Verification items for the finished model (mm, model axes). A direction names the side the tool comes from. Coordinates: 2 decimals unless noted, no trailing zeros. Write each loop counter-clockwise with the first axis right and the second up, starting at its lowest first coordinate (ties: lowest second). Pieces come first, ordered by that corner, then holes. Notation, with made-up numbers: (27, -29.5) -> (32, -29.5) arc R20 cw to (32, -22.5) -> close; hole circle Ø4 at (1, 24). An arc over 180 degrees is marked (long way). Write item = value, one per line. Start each with the question number.
(1) Gauge pin test, flat ends, axial feed: pin 1 Ø0.9 at (x, z) = (85, 1) entering from -Y; pin 2 Ø0.9 at (y, z) = (64, 1.5) entering from +X; pin 3 Ø1.5 at (y, z) = (35, 2) entering from +X. Record the tip position at first contact, or that the pin passes through.
(2) Set-up check for faces 5 (the face through (33, 63, 1)), 6 (the face through (84, 23, 1)), 7 (the face through (34.203, 6.141, 1.479)), 8 (the face through (83, 2, 1)), 9 (the face through (1, 43, 1)): record each of +Z, -Z, +X, -X, +Y, -Y from which the full face is reachable in a straight line by a thin tool's end or side.
(3) Mould release check, pull along X, two halves, no side actions. Record for faces 1 (the face through (63, 65, 1)), 2 (the face through (1, 3, 1)), 3 (the face through (43, 64, 1)), 4 (the face through (0, 1, 1)): released by +X, released by -X, zero draft, split by the parting line, or undercut.
(4) Section check D-D (y = 61.5). Record the cut outline in (x, z).
(5) Section check C-C (y = 17). Record the cut outline in (x, z), plus the area to 3 significant figures.
(6) Material ranges on probe 1 along Y at (x, z) = (42, 2.25); probe 2 along Y at (x, z) = (44, 0.2); probe 3 along X at (y, z) = (55, 2.35), recorded low to high. Write a range as [from, to].
(7) Section check A-A (x = 64). Record the cut outline in (y, z).
Autodesk Inventor part; units mm, degrees
ref_plane "YZ Plane" through (0, 0, 0) normal (1, 0, 0) x (0, 1, 0)
ref_plane "XZ Plane" through (0, 0, 0) normal (0, 1, 0) x (-1, 0, 0)
ref_plane "XY Plane" through (0, 0, 0) normal (0, 0, 1) x (1, 0, 0)
sketch "Sketch1" plane through (0, 0, 0) normal (0, 0, 1) x (1, 0, 0)
  line L0 (0, 0) -> (83, 0)
  line L1 (0, 0) -> (0, 3)
  line L2 (0, 3) -> (3, 3)
  line L3 (3, 3) -> (3, 23)
  line L4 (3, 23) -> (0, 23)
  line L5 (0, 23) -> (0, 43)
  line L6 (0, 43) -> (3, 43)
  line L7 (3, 43) -> (3, 63)
  line L8 (3, 63) -> (3, 66)
  line L9 (3, 66) -> (23, 66)
  line L10 (23, 66) -> (23, 63)
  line L11 (23, 63) -> (43, 63)
  line L12 (43, 63) -> (43, 66)
  line L13 (43, 66) -> (63, 66)
  line L14 (63, 66) -> (63, 63)
  line L15 (63, 63) -> (83, 63)
  line L16 (83, 63) -> (86, 63)
  line L17 (86, 63) -> (86, 43)
  line L18 (86, 43) -> (83, 43)
  line L19 (83, 43) -> (83, 23)
  line L20 (83, 23) -> (86, 23)
  line L21 (86, 23) -> (86, 3)
  line L22 (83, 3) -> (83, 0)
  line L23 (83, 3) -> (86, 3)
  dimension "d0" = 83
  dimension "d1" = 3
  dimension "d2" = 3
  dimension "d3" = 20
  dimension "d4" = 20
  dimension "d5" = 20
  dimension "d6" = 3
  dimension "d7" = 20
  dimension "d8" = 20
  dimension "d9" = 20
  dimension "d10" = 20
  dimension "d11" = 3
  dimension "d12" = 20
  dimension "d13" = 3
  dimension "d14" = 20
  dimension "d16" = 20
extrude "Extrusion1" add sketch "Sketch1" along normal blind 3
sketch "Sketch2" plane through (0, 0, 3) normal (0, 0, 1) x (1, 0, 0)
  line L0 (33, 20) -> (73, 20)
  line L1 (73, 20) -> (73, 5)
  line L2 (73, 5) -> (33, 5)
  line L3 (33, 5) -> (33, 20)
  line L4 (0, 0) -> (83, 0)
  line L5 (83, 23) -> (83, 43)
  dimension "d19" = 5
  dimension "d20" = 10
  dimension "d21" = 15
  dimension "d22" = 40
extrude "Extrusion2" cut sketch "Sketch2" against normal through all
fillet "Fillet1" radius 4 4 edges at (73, 5, 1.5) (73, 20, 1.5) (33, 20, 1.5) (33, 5, 1.5)
properties part number "ControlBoxSide" material "Wood (Birch)"
Response:
q1.pin_1 = 3
q1.pin_2 = 63
q1.pin_3 = 83
q2.face_5 = +Z, -Z, +Y
q2.face_6 = +Z, -Z, +X
q2.face_7 = +Z, -Z
q2.face_8 = +Z, -Z, +X, -Y
q2.face_9 = +Z, -Z, -X, +Y
q3.face_1 = released by +X
q3.face_2 = zero draft
q3.face_3 = undercut
q3.face_4 = released by -X
q4.outline = (3, 0) -> (86, 0) -> (86, 3) -> (3, 3) -> close
q5.outline = (3, 0) -> (33.13, 0) -> (33.13, 3) -> (3, 3) -> close; (72.87, 0) -> (86, 0) -> (86, 3) -> (72.87, 3) -> close
q5.area = 130 mm2
q6.probe_1 = [0, 5], [20, 63]
q6.probe_2 = [0, 5], [20, 66]
q6.probe_3 = [3, 86]
q7.outline = (0, 0) -> (5, 0) -> (5, 3) -> (0, 3) -> close; (20, 0) -> (63, 0) -> (63, 3) -> (20, 3) -> close
